The listing builds one solid part. Answer for the finished solid, in the listing's coordinates (mm). A direction names the side the tool comes from. Round coordinates to 2 decimals unless told otherwise and drop trailing zeros. Write each loop counter-clockwise with the first axis right and the second up, starting at its lowest first coordinate (ties: lowest second). Pieces come first, ordered by that corner, then holes.
Item 1: Find section B-B on z = 5. Give the number of separate pieces and of enclosed holes in the cut face, then the cut area to 3 significant figures.
Item 2: Each of these flat-tipped pins is pushed along its axis until it touches: pin 1 (5 mm diameter, centred on y = 19, z = 6.5, fed in from -X); pin 2 (4 mm diameter, centred on y = 18, z = 4.5, fed in from +X); pin 3 (4 mm diameter, centred on x = 16, z = 5, fed in from +Y); pin 4 (2 mm diameter, centred on x = 7.5, y = 15, fed in from -Z). Where does it stop, or does it pass through?
Item 3: Find the intervals of material crossed by probe 1 along Z at (x, y) = (-16, 7.75); probe 2 along X at (y, z) = (16, 4); probe 3 along Y at (x, z) = (7.5, 5.25), in increasing order.
Item 4: For a pull along X with two mould halves and no side action, classify faces 1 (the face through (-5.78, 18.64, 3.54)), 2 (the face through (0, 10, 5)), 3 (the face through (0, 26.464, 5)), 4 (the face through (-14, 16, 5)) as +X half, -X half, draft (parallel to the pull), parting line (faces both ways), or undercut.
Item 5: Find section D-D on x = 12.5. Give the vertices of the cut face in (y, z), then the cut area to 3 significant figures.
Item 6: Find section A-A on z = 0.5. Give the vertices of the cut face in (x, y), then the cut area to 3 significant figures.
Item 7: A tool of negligible diameter and unlimited length cuts with its end or side. For faces 5 (the face through (0.07, 4.93, 6.65)), 6 (the face through (-14.244, 4.443, 5.008)), 7 (the face through (0, 10, 0)), from which of +Z, -Z, +X, -X, +Y, -Y can it reach the whole face along a straight path? Write none if from no direction.
```python
from build123d import *

# Parameters (mm, degrees)
BOSS_EXTRU_1_DEPTH      = 10
ESQUISSE2_R             = 1.65
ENL_V_MAT_EXTRU_1_DEPTH = 8
ESQUISSE3_R             = 1.65
ENL_V_MAT_EXTRU_2_DEPTH = 8
CHANFREIN1_SIZE         = 5
ESQUISSE4_R             = 1.65
ENL_V_MAT_EXTRU_3_DEPTH = 10
CHANFREIN3_SIZE         = 3
ESQUISSE5_R             = 1.25
ENL_V_MAT_EXTRU_4_DEPTH = 38.754045686


with BuildPart() as part:
    # Esquisse1 → Boss.-Extru.1 (new body)
    with BuildSketch(Plane.XY):
        Polygon((-25, 0), (25, 0), (25, 5), (0, 30), (-25, 5), align=None)
    extrude(amount=BOSS_EXTRU_1_DEPTH)

    # Esquisse2 → Enlèv. mat.-Extru.1 (cut)
    with BuildSketch(Plane(origin=(15, 15, 0), x_dir=(0, 0, -1), z_dir=(0.7071067811865511, 0.7071067811865439, 0))):
        with Locations(Location((-5, 8.857864376, 0), (0, 0, 90))):
            Circle(ESQUISSE2_R)
        with Locations(Location((-5, -9.142135624, 0), (0, 0, 90))):
            Circle(ESQUISSE2_R)
    extrude(amount=-ENL_V_MAT_EXTRU_1_DEPTH, mode=Mode.SUBTRACT)

    # Esquisse3 → Enlèv. mat.-Extru.2 (cut)
    with BuildSketch(Plane(origin=(-15, 15, 0), x_dir=(0, 0, 1), z_dir=(-0.7071067811865511, 0.7071067811865439, 0))):
        with Locations(Location((5, 9.857864376, 0), (0, 0, 270))):
            Circle(ESQUISSE3_R)
        with Locations(Location((5, -8.142135624, 0), (0, 0, 270))):
            Circle(ESQUISSE3_R)
    extrude(amount=-ENL_V_MAT_EXTRU_2_DEPTH, mode=Mode.SUBTRACT)

    # Chanfrein1
    chanfrein1_edges = [part.edges().sort_by_distance(p)[0] for p in [
        (0, 30, 5),
    ]]
    chamfer(chanfrein1_edges, length=CHANFREIN1_SIZE)

    # Esquisse4 → Enlèv. mat.-Extru.3 (cut)
    with BuildSketch(Plane.XZ):
        with Locations(Location((0, 5, 0), (0, 0, 270))):
            Circle(ESQUISSE4_R)
        with Locations(Location((-16, 5, 0), (0, 0, 270))):
            Circle(ESQUISSE4_R)
        with Locations(Location((16, 5, 0), (0, 0, 90))):
            Circle(ESQUISSE4_R)
    extrude(amount=-ENL_V_MAT_EXTRU_3_DEPTH, mode=Mode.SUBTRACT)

    # Chanfrein3
    chanfrein3_edges = [part.edges().sort_by_distance(p)[0] for p in [
        (25, 0, 5),
        (-25, 0, 5),
    ]]
    chamfer(chanfrein3_edges, length=CHANFREIN3_SIZE)

    # Esquisse5 → Enlèv. mat.-Extru.4 (cut, through all)
    with BuildSketch(Plane.XY.offset(10)):
        with Locations((7.5, 15)):
            Circle(ESQUISSE5_R)
        with Locations((7.5, 5)):
            Circle(ESQUISSE5_R)
    extrude(amount=-ENL_V_MAT_EXTRU_4_DEPTH, mode=Mode.SUBTRACT)


solid = part.part
```
Check values:
1. separate pieces: 3
1. enclosed holes: 2
1. area: 659 mm2
2. pin 1: stops at x = -13.5
2. pin 2: stops at x = 14
2. pin 3: stops at y = 16
2. pin 4: passes through
3. probe 1: z = 0 to 3.35, 6.65 to 10
3. probe 2: x = -14 to -3.91, -2.69 to 2.69, 5.33 to 6.75, 8.25 to 14
3. probe 3: y = 0 to 3.75, 6.25 to 13.75, 16.25 to 17.72, 22.33 to 22.5
4. face 1: undercut
4. face 2: undercut
4. face 3: draft
4. face 4: -X half
5. outline: (0, 0) - (17.5, 0) - (17.5, 10) - (0, 10) - close
5. area: 175 mm2
6. outline: (-25, 3) - (-22, 0) - (22, 0) - (25, 3) - (25, 5) - (3.54, 26.46) - (-3.54, 26.46) - (-25, 5) - close; hole circle Ø2.5 at (7.5, 5); hole circle Ø2.5 at (7.5, 15)
6. area: 844 mm2
7. face 5: -Y
7. face 6: none
7. face 7: -Z, +X, -X, +Y, -Y
